Read the model definition and answer for the solid it produces. Units are mm, in the model's axes. A direction names the side the tool comes from. Give positions to 0.01 mm unless a question says otherwise; leave off trailing zeros. Write each loop counter-clockwise with the first axis right and the second up, starting at its lowest first coordinate (ties: lowest second). Pieces come first, ordered by that corner, then holes. Notation, with made-up numbers: (47.25, 79.25) - (94.25, 79.25) arc R16 cw to (94.25, 90.25) - close; hole circle Ø7 at (-31.5, 61). An arc over 180 degrees is marked (long way). Answer as CSV lines item,"result".
```python
from build123d import *

# Parameters (mm, degrees)
BOSS_EXTRUDE1_DEPTH        = 80
SKETCH2_W                  = 20
SKETCH2_H                  = 10
CUT_EXTRUDE1_DEPTH         = 209
SKETCH3_R                  = 10
CUT_EXTRUDE2_DEPTH         = 40
BOSS_EXTRUDE2_START        = 10
SKETCH4_R                  = 20
SKETCH4_R_2                = 10
BOSS_EXTRUDE2_DEPTH        = 10
F_20_0MM_DOWEL_HOLE1_D     = 20
F_20_0MM_DOWEL_HOLE1_DEPTH = 50
F_20_0MM_DOWEL_HOLE1_TIP   = 6.00860619
CUT_EXTRUDE3_DEPTH         = 20
SKETCH10_R                 = 10
CUT_EXTRUDE4_DEPTH         = 74
SKETCH11_R                 = 25
SKETCH11_R_2               = 10
CUT_EXTRUDE5_DEPTH         = 40
SKETCH12_R                 = 25
CUT_EXTRUDE6_DEPTH         = 10
SKETCH14_R                 = 35
SKETCH14_R_2               = 25
CUT_EXTRUDE7_DEPTH         = 30
SKETCH15_R                 = 35
CUT_EXTRUDE8_DEPTH         = 30
CUT_EXTRUDE9_DEPTH         = 20
BOSS_EXTRUDE3_START        = 25
SKETCH17_W                 = 20
SKETCH17_H                 = 5
BOSS_EXTRUDE3_DEPTH        = 25
SKETCH18_W                 = 20
SKETCH18_H                 = 5
BOSS_EXTRUDE4_DEPTH        = 25
SKETCH19_W                 = 20
SKETCH19_H                 = 5
BOSS_EXTRUDE5_DEPTH        = 25
CHAMFER1_SIZE2             = 20
CHAMFER1_SIZE              = 25
CHAMFER3_SIZE2             = 25
CHAMFER3_SIZE              = 20


with BuildPart() as part:
    # Sketch1 → Boss-Extrude1 (new body)
    with BuildSketch(Plane.XY):
        with BuildLine():
            ThreePointArc((0, 50), (14.644660941, 14.644660941), (50, 0))
            Line((50, 0), (130, 0))
            ThreePointArc((130, 0), (165.355339059, 14.644660941), (180, 50))
            ThreePointArc((180, 50), (165.355339059, 85.355339059), (130, 100))
            Line((130, 100), (50, 100))
            ThreePointArc((50, 100), (14.644660941, 85.355339059), (0, 50))
        make_face()
    extrude(amount=BOSS_EXTRUDE1_DEPTH)

    # Sketch2 → Cut-Extrude1 (cut)
    with BuildSketch(Plane(origin=(0, 0, 0), x_dir=(0, 0, -1), z_dir=(1, 0, 0))):
        with Locations((-70, 75)):
            Rectangle(SKETCH2_W, SKETCH2_H)
        with Locations((-70, 25)):
            Rectangle(SKETCH2_W, SKETCH2_H)
    extrude(amount=CUT_EXTRUDE1_DEPTH, mode=Mode.SUBTRACT)

    # Sketch3 → Cut-Extrude2 (cut)
    with BuildSketch(Plane.XY.offset(80)):
        with Locations((130, 50)):
            Circle(SKETCH3_R)
    extrude(amount=-CUT_EXTRUDE2_DEPTH, mode=Mode.SUBTRACT)

    # Sketch4 → Boss-Extrude2 (add)
    with BuildSketch(Plane.XY.offset(80).offset(BOSS_EXTRUDE2_START)):
        with Locations(Location((130, 50, 0), (0, 0, 270))):
            Circle(SKETCH4_R)
        with Locations((130, 50)):
            Circle(SKETCH4_R_2, mode=Mode.SUBTRACT)
    extrude(amount=-BOSS_EXTRUDE2_DEPTH)

    # Ø20.0mm Dowel Hole1
    with Locations(Plane(origin=(130, 50, 90), x_dir=(1, 0, 0), z_dir=(0, 0, 1))):
        with Locations((0, 0)):
            Hole(F_20_0MM_DOWEL_HOLE1_D / 2, depth=F_20_0MM_DOWEL_HOLE1_DEPTH)
            with Locations((0, 0, -(F_20_0MM_DOWEL_HOLE1_DEPTH + F_20_0MM_DOWEL_HOLE1_TIP / 2))):  # 118° drill point
                Cone(0, F_20_0MM_DOWEL_HOLE1_D / 2, F_20_0MM_DOWEL_HOLE1_TIP, mode=Mode.SUBTRACT)

    # Sketch9 → Cut-Extrude3 (cut)
    with BuildSketch(Plane.XY.offset(80)):
        with BuildLine():
            Line((130, 70), (4.17424305, 70))
            ThreePointArc((4.17424305, 70), (0, 50), (4.17424305, 30))
            Line((4.17424305, 30), (130, 30))
            ThreePointArc((130, 30), (110, 50), (130, 70))
        make_face()
    extrude(amount=-CUT_EXTRUDE3_DEPTH, mode=Mode.SUBTRACT)

    # Sketch10 → Cut-Extrude4 (cut)
    with BuildSketch(Plane.XY.offset(60)):
        with Locations((50, 50)):
            Circle(SKETCH10_R)
    extrude(amount=-CUT_EXTRUDE4_DEPTH, mode=Mode.SUBTRACT)

    # Sketch11 → Cut-Extrude5 (cut)
    with BuildSketch(Plane.XY.offset(60)):
        with Locations((50, 50)):
            Circle(SKETCH11_R)
        with Locations((50, 50)):
            Circle(SKETCH11_R_2, mode=Mode.SUBTRACT)
    extrude(amount=-CUT_EXTRUDE5_DEPTH, mode=Mode.SUBTRACT)

    # Sketch12 → Cut-Extrude6 (cut)
    with BuildSketch(Plane.XY.offset(60)):
        with BuildLine():
            Line((70, 80), (10, 80))
            ThreePointArc((10, 80), (0, 50), (10, 20))
            Line((10, 20), (70, 20))
            ThreePointArc((70, 20), (86.055512755, 50), (70, 80))
        make_face()
        with Locations((50, 50)):
            Circle(SKETCH12_R, mode=Mode.SUBTRACT)
    extrude(amount=-CUT_EXTRUDE6_DEPTH, mode=Mode.SUBTRACT)

    # Sketch14 → Cut-Extrude7 (cut)
    with BuildSketch(Plane.XY.offset(60)):
        with Locations((50, 50)):
            Circle(SKETCH14_R)
        with Locations((50, 50)):
            Circle(SKETCH14_R_2, mode=Mode.SUBTRACT)
    extrude(amount=-CUT_EXTRUDE7_DEPTH, mode=Mode.SUBTRACT)

    # Sketch15 → Cut-Extrude8 (cut)
    with BuildSketch(Plane.XY.offset(80)):
        with Locations((50, 50)):
            Circle(SKETCH15_R)
    extrude(amount=-CUT_EXTRUDE8_DEPTH, mode=Mode.SUBTRACT)

    # Sketch16 → Cut-Extrude9 (cut)
    with BuildSketch(Plane.XY.offset(80)):
        with BuildLine():
            Line((130, 70), (175.82575695, 70))
            ThreePointArc((175.82575695, 70), (180, 50), (175.82575695, 30))
            Line((175.82575695, 30), (130, 30))
            ThreePointArc((130, 30), (150, 50), (130, 70))
        make_face()
    extrude(amount=-CUT_EXTRUDE9_DEPTH, mode=Mode.SUBTRACT)

    # Sketch17 → Boss-Extrude3 (add)
    with BuildSketch(Plane.XY.offset(60).offset(BOSS_EXTRUDE3_START)):
        with BuildLine():
            Line((150, 45), (150, 50))
            ThreePointArc((150, 50), (149.840593925, 47.47991415), (149.364916731, 45))
            Line((149.364916731, 45), (150, 45))
        make_face()
        with Locations((160, 47.5)):
            Rectangle(SKETCH17_W, SKETCH17_H)
        with BuildLine():
            ThreePointArc((110.635083269, 45), (110.159406075, 47.47991415), (110, 50))
            Line((110, 50), (110, 45))
            Line((110, 45), (110.635083269, 45))
        make_face()
        with Locations((100, 47.5)):
            Rectangle(SKETCH17_W, SKETCH17_H)
    extrude(amount=-BOSS_EXTRUDE3_DEPTH)

    # Sketch18 → Boss-Extrude4 (add)
    with BuildSketch(Plane.XY.offset(85)):
        with BuildLine():
            ThreePointArc((110.635083269, 55), (110.159406075, 52.52008585), (110, 50))
            Line((110, 50), (110, 55))
            Line((110, 55), (110.635083269, 55))
        make_face()
        with Locations((100, 52.5)):
            Rectangle(SKETCH18_W, SKETCH18_H)
    extrude(amount=-BOSS_EXTRUDE4_DEPTH)

    # Sketch19 → Boss-Extrude5 (add)
    with BuildSketch(Plane.XY.offset(85)):
        with BuildLine():
            Line((150, 55), (149.364916731, 55))
            ThreePointArc((149.364916731, 55), (149.840593925, 52.52008585), (150, 50))
            Line((150, 50), (150, 55))
        make_face()
        with Locations((160, 52.5)):
            Rectangle(SKETCH19_W, SKETCH19_H)
    extrude(amount=-BOSS_EXTRUDE5_DEPTH)

    # Chamfer1
    chamfer1_edges = [part.edges().sort_by_distance(p)[0] for p in [
        (90, 52.5, 85),
    ]]
    chamfer1_side = [part.faces().sort_by_distance(p)[0] for p in [
        (90, 52.5, 84.6),
    ]]
    chamfer(chamfer1_edges, length=CHAMFER1_SIZE - 0.0001, length2=CHAMFER1_SIZE2 - 0.0001, reference=chamfer1_side[0])  # a hair under: the kernel refuses the full size

    # Chamfer3
    chamfer3_edges = [part.edges().sort_by_distance(p)[0] for p in [
        (170, 52.5, 85),
    ]]
    chamfer3_side = [part.faces().sort_by_distance(p)[0] for p in [
        (169.6, 52.5, 85),
    ]]
    chamfer(chamfer3_edges, length=CHAMFER3_SIZE - 0.0001, length2=CHAMFER3_SIZE2 - 0.0001, reference=chamfer3_side[0])  # a hair under: the kernel refuses the full size


solid = part.part
```
(1) Each of these flat-tipped pins is pushed along its axis until it touches: P1, Ø24, axis at x = 21.5, z = 60, coming from the +Y side; P2, Ø10, axis at y = 32, z = 52, coming from the -X side; P3, Ø5, axis at y = 23.5, z = 20, coming from the +X side. Where does it stop, or does it pass through?
Worked out:
P1,"stops at y = 97.2"
P2,"stops at x = 1.83"
P3,"stops at x = 173.86"
(2) A cutting plane is placed at C-C (y = 32). Write down the section's boundary in (x, z), and give its area (3 significant figures).
Worked out:
outline,"(3.35, 0) - (176.65, 0) - (176.65, 60) - (138.72, 60) - (138.72, 90) - (121.28, 90) - (121.28, 60) - (81.24, 60) - (81.24, 50) - (80.02, 50) - (80.02, 30) - (67.35, 30) - (67.35, 20) - (32.65, 20) - (32.65, 30) - (19.98, 30) - (19.98, 50) - (3.35, 50) - close"
area,"8,590 mm^2"
(3) Find the intervals of material crossed by L1, parallel to X at y = 50, z = 41; L2, parallel to Y at x = 110, z = 66; L3, parallel to Y at x = 50, z = 23, in increasing order.
Worked out:
L1,"x = 0 to 15, 85 to 120, 140 to 180"
L2,"y = 0 to 20, 45 to 55, 80 to 100"
L3,"y = 0 to 25, 75 to 100"
(4) For faces 4 (the flat face through (103, 55, 70)), 5 (the flat face through (89, 90, 80)), 6 (the flat face through (157, 45, 70)), 7 (the flat face through (89, 10, 80)), determine the directions among +Z, -Z, +X, -X, +Y, -Y from which every point of the face is accessible in a straight line to the end or side of a thin tool.
Worked out:
face 4,"+Z, -X"
face 5,"+Z, +X, -X, +Y"
face 6,"+Z, +X"
face 7,"+Z, +X, -X, -Y"
(5) A cutting plane is placed at B-B (x = 27.5). Write down the section's boundary in (y, z).
Worked out:
outline,"(5.35, 0) - (94.65, 0) - (94.65, 80) - (80, 80) - (80, 50) - (76.81, 50) - (76.81, 30) - (60.9, 30) - (60.9, 20) - (39.1, 20) - (39.1, 30) - (23.19, 30) - (23.19, 50) - (20, 50) - (20, 80) - (5.35, 80) - close"
(6) A cutting plane is placed at A-A (z = 47). Write down the section's boundary in (x, y), and give its area (3 significant figures).
Worked out:
outline,"(50, 0) - (130, 0) arc R50 ccw to (130, 100) - (50, 100) arc R50 ccw to start; hole circle Ø70 at (50, 50); hole circle Ø20 at (130, 50)"
area,"11,700 mm^2"
(7) A cutting plane is placed at D-D (x = 159). Write down the section's boundary in (y, z), and give its area (3 significant figures).
Worked out:
outline,"(9.27, 0) - (90.73, 0) - (90.73, 80) - (80, 80) - (80, 60) - (55, 60) - (55, 73.75) - (45, 73.75) - (45, 60) - (20, 60) - (20, 80) - (9.27, 80) - close"
area,"5,450 mm^2"
(8) The mould has two halves that part along X. Classify faces 1 (the cylindrical face through (127.83, 40.24, 65.35)), 2 (the flat face through (85.7, 50.1, 50)), 3 (the cylindrical face through (122.34, 31.525, 75.21)): +X half, -X half, draft (parallel to the pull), parting line (faces both ways), or undercut.
Worked out:
face 1,"undercut"
face 2,"draft"
face 3,"parting line"
